Autodesk Fusion 360 part; units mm, degrees
sketch "Sketch1" plane through (0, 0, 0) normal (0, 0, 1) x (1, 0, 0)
  line L0 (0, 0) -> (47.5, 0)
  line L1 (47.5, 0) -> (47.5, 26)
  line L2 (47.5, 26) -> (0, 26)
  line L3 (0, 26) -> (0, 0)
  circle A0 centre (6, 21) radius 1.5
  circle A1 centre (43, 5) radius 1.5
  dimension "d1" = 47.5
  dimension "d2" = 26
  dimension "d3" = 3
  dimension "d4" = 3
  dimension "d5" = 5
  dimension "d6" = 6
  dimension "d7" = 4.5
  dimension "d8" = 5
  dimension "d103" = 0
  dimension "d104" = 0
  dimension "d105" = 0
  dimension "d106" = 0
  dimension "d127" = 0
  dimension "d128" = 0
  dimension "d129" = 0
  dimension "d130" = 0
extrude "Extrude1" add sketch "Sketch1" along normal blind 1
sketch "Sketch2" plane through (0, 0, 1) normal (0, 0, 1) x (-1, 0, 0)
  circle A0 centre (-43, -5) radius 1.5
  circle A1 centre (-6, -21) radius 1.5
  line L0 (0, -26) -> (0, 0)
  line L1 (0, 0) -> (-47.5, 0)
  line L2 (-47.5, 0) -> (-47.5, -26)
  line L3 (-47.5, -26) -> (0, -26)
  circle A2 centre (-30, -12) radius 10.2956
  circle A3 centre (-30, -12) radius 8.6023
  dimension "d13" = 30
extrude "Extrude2" add sketch "Sketch2" along normal blind 3 contours A2
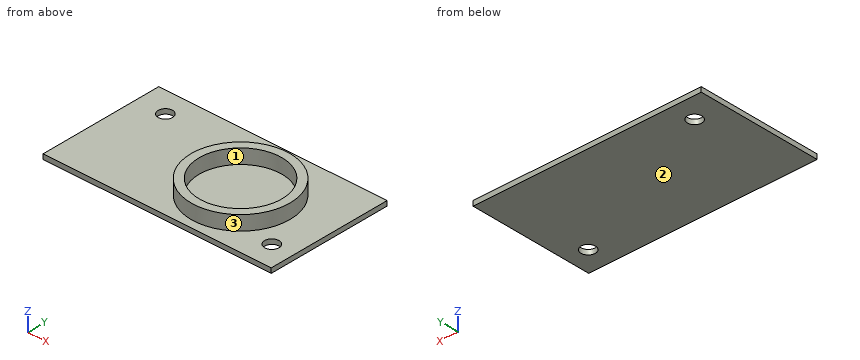
Design review of the part built by this model. Coordinates are the model's own, in mm. Face numbers are marked on the shaded views. Round coordinates to 2 decimals unless told otherwise and drop trailing zeros. Write each loop counter-clockwise with the first axis right and the second up, starting at its lowest first coordinate (ties: lowest second). Pieces come first, ordered by that corner, then holes. Notation, with made-up numbers: (-12, 57.5) -> (13, 57.5) arc R21 ccw to (13, 88.5) -> close; hole circle Ø11 at (51.25, 77.25). An arc over 180 degrees is marked (long way). Write item = value, one per line. Start each with the question number.
1) Mouldability with a two-part tool opening along Y and no side actions: class the marked faces 1, 2 and 3 as +Y half, -Y half, draft (parallel to the pull), parting line (faces both ways), or undercut.
2) Take a section at D-D, the plane x = 42.5. State the section outline as (y, z) points, plus the area to 3 significant figures.
3) Clearance check with flat-ended pins moving along their axes: pin 1 (1 mm diameter, centred on y = 15.5, z = 3.5, fed in from -X); pin 2 (4 mm diameter, centred on x = 43, y = 5, fed in from -Z). State where each tip first meets the part, or that it passes through.
4) Take a section at A-A, the plane x = 6. State the section outline as (y, z) points.
5) Wall thickness on probe 1 along Y at (x, z) = (43, 0.65); probe 2 along Y at (x, z) = (30, 2.6); probe 3 along X at (y, z) = (12, 2.45): over which ranges is each line inside the solid? List them lowest first. Write a range as from..to.
6) Take a section at B-B, the plane y = 12. State the section outline as (x, z) points.
7) Take a section at C-C, the plane z = 2.8. State the section outline as (x, y) points.
Results list:
q1.face_1 = undercut
q1.face_2 = draft
q1.face_3 = parting line
q2.outline = (0, 0) -> (3.59, 0) -> (3.59, 1) -> (0, 1) -> close; (6.41, 0) -> (26, 0) -> (26, 1) -> (6.41, 1) -> close
q2.area = 23.2 mm²
q3.pin_1 = 20.15
q3.pin_2 = 0
q4.outline = (0, 0) -> (19.5, 0) -> (19.5, 1) -> (0, 1) -> close; (22.5, 0) -> (26, 0) -> (26, 1) -> (22.5, 1) -> close
q5.probe_1 = 0..3.5, 6.5..26
q5.probe_2 = 1.7..3.4, 20.6..22.3
q5.probe_3 = 19.7..21.4, 38.6..40.3
q6.outline = (0, 0) -> (47.5, 0) -> (47.5, 1) -> (40.3, 1) -> (40.3, 4) -> (38.6, 4) -> (38.6, 1) -> (21.4, 1) -> (21.4, 4) -> (19.7, 4) -> (19.7, 1) -> (0, 1) -> close
q7.outline = circle Ø20.59 at (30, 12); hole circle Ø17.2 at (30, 12)
